from build123d import *

# Parameters (mm, degrees)
F0_R     = 4.25
F1_DEPTH = 3
F2_R     = 2.5
F3_DEPTH = 1.5
F6_W     = 3
F6_H     = 3
F7_DEPTH = 25
F8_COUNT = 4
F10_R    = 0.5


with BuildPart() as f1:
    # F0 (on Top) → F1 (new body)
    with BuildSketch(Plane.XY):
        Circle(F0_R)
    extrude(amount=F1_DEPTH)

    # F2 (on face) → F3 (join)
    with BuildSketch(Plane.XY.offset(3)):
        Circle(F2_R)
    extrude(amount=F3_DEPTH)

    # F4 (on Right) → F5 (revolve)
    with BuildSketch(Plane.YZ):
        with BuildLine():
            Line((-2.5, 4.5), (0, 4.5))
            Line((0, 4.5), (0, 7))
            ThreePointArc((0, 7), (-1.767766953, 6.267766953), (-2.5, 4.5))
        make_face()
    revolve(axis=Axis((0, 0, 5.75), (0, 0, -1)))


with BuildPart() as f7:
    # F6 (on face) → F7 (new body)
    with BuildSketch(Plane.XY.offset(4.5)):
        with Locations((2, -2)):
            Rectangle(F6_W, F6_H)
    extrude(amount=F7_DEPTH)


with BuildPart() as f8_1:
    # F8: instance of F7
    add(f7.part.rotate(Axis((0, 0, 5.75), (0, 0, -1)), 1 * 360 / F8_COUNT))


with BuildPart() as f8_2:
    # F8: instance of F7
    add(f7.part.rotate(Axis((0, 0, 5.75), (0, 0, -1)), 2 * 360 / F8_COUNT))


with BuildPart() as f8_3:
    # F8: instance of F7
    add(f7.part.rotate(Axis((0, 0, 5.75), (0, 0, -1)), 3 * 360 / F8_COUNT))


with BuildPart() as f1_1:
    add(f1.part)

    # F9: cut F8_1, F8_2, F8_3, F7
    add(f8_1.part, mode=Mode.SUBTRACT)
    add(f8_2.part, mode=Mode.SUBTRACT)
    add(f8_3.part, mode=Mode.SUBTRACT)
    add(f7.part, mode=Mode.SUBTRACT)

    # F10
    f10_edges = [f1_1.edges().sort_by_distance(p)[0] for p in [
        (-4.25, 0, 3),
        (-4.25, 0, 0),
        (-2.5, 0, 3),
    ]]
    fillet(f10_edges, radius=F10_R)


solid = f1_1.part
Model file for the job. Use its own axes, mm. A direction names the side the tool comes from. Give positions to 0.01 mm unless a question says otherwise; leave off trailing zeros. Order: outer loops, then holes, each group sorted by start corner. A loop starts at its lowest first (then second) coordinate and runs counter-clockwise, first axis right, second up. Notation, with made-up numbers: (7.5, -4.75) - (55.5, -4.75) arc R22 ccw to (55.5, 24.25) - close; hole circle Ø9 at (27.25, 24). An arc over 180 degrees is marked (long way). Return JSON: item names as keys, results as strings.
1) Cut at C-C, the plane z = 1.5. Give the cut face in (x, y), plus the area to 3 significant figures.
Geometry says:
{"outline": "circle Ø8.5 at (0, 0)", "area": "56.7 mm²"}
2) 3-axis set-ups, long thin cutter, end or side, ignore diameter. For faces 1 (the flat face through (-1, 0.5, 5)), 2 (the flat face through (0.5, -1, 5)), 3 (the flat face through (1, 3, 3)), 4 (the flat face through (-0.5, -1, 5)), 5 (the flat face through (0.5, 1, 5)): which of +Z, -Z, +X, -X, +Y, -Y reach the whole face in a straight line?
Geometry says:
{"face 1": "+Z, -X, +Y", "face 2": "+Z, +X, -Y", "face 3": "+Z", "face 4": "+Z, -X, -Y", "face 5": "+Z, +X, +Y"}
3) Cut at A-A, the plane y = 0. Give the cut face in (x, z), plus the area to 3 significant figures.
Geometry says:
{"outline": "(-4.25, 0.5) arc R0.5 ccw to (-3.75, 0) - (3.75, 0) arc R0.5 ccw to (4.25, 0.5) - (4.25, 2.5) arc R0.5 ccw to (3.75, 3) - (3, 3) arc R0.5 cw to (2.5, 3.5) - (2.5, 4.5) arc R2.5 ccw to (-2.5, 4.5) - (-2.5, 3.5) arc R0.5 cw to (-3, 3) - (-3.75, 3) arc R0.5 ccw to (-4.25, 2.5) - close", "area": "42.7 mm²"}
4) Flat gauge pins, fed straight in: P1, Ø1, axis at x = -2, y = -1.5, coming from the +Z side; P2, Ø1.6, axis at y = -1.5, z = 5.5, coming from the -X side; P3, Ø1.6, axis at y = 1.5, z = 5.5, coming from the +X side. Where does each tip first touch, or does it go through?
Geometry says:
{"P1": "z = 4.5", "P2": "x = -0.5", "P3": "x = 0.5"}
5) Cut at D-D, the plane z = 5. Give the cut face in (x, y).
Geometry says:
{"outline": "(-2.4, -0.5) - (-0.5, -0.5) - (-0.5, -2.4) arc R2.45 ccw to (0.5, -2.4) - (0.5, -0.5) - (2.4, -0.5) arc R2.45 ccw to (2.4, 0.5) - (0.5, 0.5) - (0.5, 2.4) arc R2.45 ccw to (-0.5, 2.4) - (-0.5, 0.5) - (-2.4, 0.5) arc R2.45 ccw to start"}
6) Probe line 1 (Z direction, x = -1.5, y = -0.75); line 2 (Z direction, x = 2.25, y = -2.75); line 3 (Y direction, x = -2.25, z = 5). List the from-to ranges inside material, lowest first. Write a range as from..to.
Geometry says:
{"line 1": "0..4.5", "line 2": "0..3", "line 3": "-0.5..0.5"}
